Autodesk Inventor part; units mm, degrees
ref_plane "YZ Plane" through (0, 0, 0) normal (1, 0, 0) x (0, 1, 0)
ref_plane "XZ Plane" through (0, 0, 0) normal (0, 1, 0) x (-1, 0, 0)
ref_plane "XY Plane" through (0, 0, 0) normal (0, 0, 1) x (1, 0, 0)
sketch "Sketch1" plane through (0, 0, 0) normal (0, 1, 0) x (-1, 0, 0)
  arc A0 (0, 6.5) -> (0, -6.5) centre (0, 0) ccw
  arc A1 (17.43, -3.75) -> (17.43, 3.75) centre (17.43, 0) ccw
  line L0 (10.43, 3.75) -> (17.43, 3.75)
  line L1 (10.43, -3.75) -> (17.43, -3.75)
  line L2 (0, 0) -> (20.86, 0) construction
  circle A2 centre (0, 0) radius 2.75
  circle A3 centre (17.43, 0) radius 1.5
  circle A4 centre (10.43, 0) radius 1.5
  line L3 (10.43, 3.75) -> (0, 6.5)
  line L4 (10.43, -3.75) -> (0, -6.5)
  line L5 (10.43, 0) -> (10.43, -12.3931) construction
  line L6 (0, 8.169) -> (0, -9.3531) construction
  dimension "d0" = 13
  dimension "d1" = 7.5
  dimension "d2" = 17.43
  dimension "d3" = 7.5
  dimension "d6" = 0
  dimension "d7" = 3.75
  dimension "d8" = 5.5
  dimension "d10" = 3
  dimension "d11" = 3
  dimension "d14" = 7
  dimension "d17" = 17.43
  dimension "d20" = 0
  dimension "d21" = 0
  dimension "d22" = 0
  dimension "d23" = 0
  dimension "d24" = 0
extrude "Extrusion1" add sketch "Sketch1" along normal blind 6
fillet "Fillet1" radius 5 1 edges at (-10.43, 3, 3.75)
fillet "Fillet2" radius 5 1 edges at (-10.43, 3, -3.75)
fillet "Fillet3" radius 5 2 edges at (0, 3, -6.5) (0, 3, 6.5)
properties part number "adaptator_25"
Read the model definition and answer for the solid it produces. Units are mm, in the model's axes. A direction names the side the tool comes from. Coordinates: 2 decimals unless noted, no trailing zeros. Loops run counter-clockwise (first coordinate to the right, second up) from the corner with the lowest first, then second, coordinate; pieces in that order, holes last. Notation, with made-up numbers: (41.25, -36.5) - (46.25, -36.5) arc R31 ccw to (46.25, 2.5) - close; hole circle Ø4 at (59, 78). An arc over 180 degrees is marked (long way). Answer in a Markdown table with one row per item.
1. Find section A-A, the plane y = 0.8. Write down the section's boundary in (x, z), then the cut area to 3 significant figures.
Conclusion:
| item | result |
|---|---|
| outline | (-17.43, -3.75) - (-11.08, -3.75) arc R5 cw to (-9.8, -3.92) - (-0.85, -6.27) arc R5 ccw to (1.82, -6.24) arc R6.5 ccw to (1.82, 6.24) arc R5 ccw to (-0.85, 6.27) - (-9.8, 3.92) arc R5 cw to (-11.08, 3.75) - (-17.43, 3.75) arc R3.75 ccw to start; hole circle Ø3 at (-17.43, 0); hole circle Ø3 at (-10.43, 0); hole circle Ø5.5 at (0, 0) |
| area | 210 mm² |
2. Straight lines are drawn through the part: line 1 (Z direction, x = -17.43, y = 3.4); line 2 (Z direction, x = 0, y = 2.5); line 3 (X direction, y = 1.2, z = 0.5). For each, find the intervals that lie inside material, in ascending order.
Conclusion:
| item | result |
|---|---|
| line 1 | z = -3.75 to -1.5, 1.5 to 3.75 |
| line 2 | z = -6.42 to -2.75, 2.75 to 6.42 |
| line 3 | x = -21.15 to -18.84, -16.02 to -11.84, -9.02 to -2.7, 2.7 to 6.48 |
3. Determine the mould class of faces 1 (the face through (0.596, 2.958, 2.685)), 2 (the face through (-10.426, 3.042, 3.793)), 3 (the face through (-10.44, 3.04, -3.79)) for opening direction Z: +Z half, -Z half, draft (parallel to the pull), parting line (faces both ways), or undercut.
Conclusion:
| item | result |
|---|---|
| face 1 | undercut |
| face 2 | +Z half |
| face 3 | -Z half |
4. Find section B-B, the plane z = 0. Write down the section's boundary in (x, y).
Conclusion:
| item | result |
|---|---|
| outline | (-21.18, 0) - (-18.93, 0) - (-18.93, 6) - (-21.18, 6) - close; (-15.93, 0) - (-11.93, 0) - (-11.93, 6) - (-15.93, 6) - close; (-8.93, 0) - (-2.75, 0) - (-2.75, 6) - (-8.93, 6) - close; (2.75, 0) - (6.5, 0) - (6.5, 6) - (2.75, 6) - close |
5. Find section D-D, the plane x = 0. Write down the section's boundary in (y, z).
Conclusion:
| item | result |
|---|---|
| outline | (0, -6.42) - (6, -6.42) - (6, -2.75) - (0, -2.75) - close; (0, 2.75) - (6, 2.75) - (6, 6.42) - (0, 6.42) - close |
6. Given pin 1 (1.5 mm diameter, centred on x = -7.5, y = 3, fed in from +Z); pin 2 (4 mm diameter, centred on x = -10.43, z = 0, fed in from +Y); pin 3 (2.5 mm diameter, centred on x = -17.43, z = 0, fed in from +Y); pin 4 (1.5 mm diameter, centred on y = 0.5, z = 1, fed in from -X), each flat-ended and moving along its own axis, determine where each tip first touches the part or whether it passes through.
Conclusion:
| item | result |
|---|---|
| pin 1 | stops at z = 4.72 |
| pin 2 | stops at y = 6 |
| pin 3 | passes through |
| pin 4 | stops at x = -21.17 |
7. Which of the six approach directions +Z, -Z, +X, -X, +Y, -Y give full straight-line access (tool end or side, diameter ignored) to faces 4 (the face through (-7, 6, 0)), 5 (the face through (-14, 3, 3.75)), 6 (the face through (-14, 3, -3.75))?
Conclusion:
| item | result |
|---|---|
| face 4 | +Z, -Z, +X, -X, +Y |
| face 5 | +Z, -X, +Y, -Y |
| face 6 | -Z, -X, +Y, -Y |
8. Find section C-C, the plane x = -11.5. Write down the section's boundary in (y, z).
Conclusion:
| item | result |
|---|---|
| outline | (0, -3.75) - (6, -3.75) - (6, -1.05) - (0, -1.05) - close; (0, 1.05) - (6, 1.05) - (6, 3.75) - (0, 3.75) - close |
